Can you work these out from the model? Positions are in its coordinate system, mm. Coordinates: 2 decimals unless noted, no trailing zeros. Write each loop counter-clockwise with the first axis right and the second up, starting at its lowest first coordinate (ties: lowest second). Pieces come first, ordered by that corner, then holes. Notation, with made-up numbers: M 60,-35.5 L 75,-35.5 A18 cw 75,-26.5 Z; hole C 78.25,42.25 d6. An arc over 180 degrees is marked long. Answer as a JSON object with one key per item and string values. Group by question number.
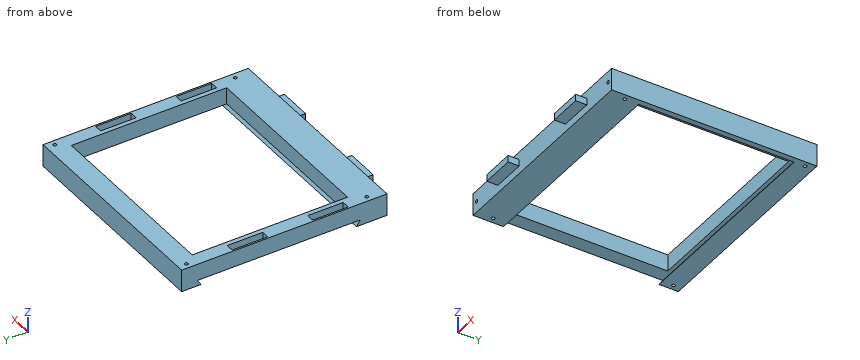
from build123d import *

# Parameters (mm, degrees)
ESBO_O1_W                = 195
ESBO_O1_H                = 185
RESSALTO_EXTRUS_O1_DEPTH = 20
ESBO_O2_W                = 30
ESBO_O2_H                = 6
RESSALTO_EXTRUS_O2_DEPTH = 10
ESBO_O3_W                = 7
ESBO_O3_H                = 32
CORTE_EXTRUS_O1_DEPTH    = 10
ESBO_O5_R                = 1.5
CORTE_EXTRUS_O3_DEPTH    = 8
ESBO_O6_R                = 1.5
CORTE_EXTRUS_O4_DEPTH    = 21
ESBO_O8_W                = 170
ESBO_O8_H                = 140
CORTE_EXTRUS_O6_DEPTH    = 21
CORTE_EXTRUS_O7_DEPTH    = 190


with BuildPart() as part:
    # Esboço1 → Ressalto-extrusão1 (new body)
    with BuildSketch(Plane.XY):
        Rectangle(ESBO_O1_W, ESBO_O1_H)
    extrude(amount=RESSALTO_EXTRUS_O1_DEPTH)

    # Esboço2 → Ressalto-extrusão2 (add)
    with BuildSketch(Plane.XZ.offset(92.5)):
        with Locations((-47.5, 10)):
            Rectangle(ESBO_O2_W, ESBO_O2_H)
        with Locations((47.5, 10)):
            Rectangle(ESBO_O2_W, ESBO_O2_H)
    extrude(amount=RESSALTO_EXTRUS_O2_DEPTH)

    # Esboço3 → Corte-extrusão1 (cut)
    with BuildSketch(Plane.XY.offset(20)):
        with Locations((-92.5, 30)):
            Rectangle(ESBO_O3_W, ESBO_O3_H)
        with Locations((-92.5, -42.5)):
            Rectangle(ESBO_O3_W, ESBO_O3_H)
        with Locations((92.5, -42.5)):
            Rectangle(ESBO_O3_W, ESBO_O3_H)
        with Locations((92.5, 30)):
            Rectangle(ESBO_O3_W, ESBO_O3_H)
    extrude(amount=-CORTE_EXTRUS_O1_DEPTH, mode=Mode.SUBTRACT)

    # Esboço5 → Corte-extrusão3 (cut)
    with BuildSketch(Plane.XZ.offset(92.5)):
        with Locations((-92.5, 10)):
            Circle(ESBO_O5_R)
        with Locations((92.5, 10)):
            Circle(ESBO_O5_R)
    extrude(amount=-CORTE_EXTRUS_O3_DEPTH, mode=Mode.SUBTRACT)

    # Esboço6 → Corte-extrusão4 (cut, through all)
    with BuildSketch(Plane(origin=(0, 0, 0), x_dir=(-1, 0, 0), z_dir=(0, 0, -1))):
        with Locations((-92.5, 85)):
            Circle(ESBO_O6_R)
        with Locations((92.5, 85)):
            Circle(ESBO_O6_R)
        with Locations((-92.5, -77.5)):
            Circle(ESBO_O6_R)
        with Locations((92.5, -77.5)):
            Circle(ESBO_O6_R)
    extrude(amount=-CORTE_EXTRUS_O4_DEPTH, mode=Mode.SUBTRACT)

    # Esboço8 → Corte-extrusão6 (cut, through all)
    with BuildSketch(Plane(origin=(0, 0, 0), x_dir=(-1, 0, 0), z_dir=(0, 0, -1))):
        with Locations((0, 5)):
            Rectangle(ESBO_O8_W, ESBO_O8_H)
    extrude(amount=-CORTE_EXTRUS_O6_DEPTH, mode=Mode.SUBTRACT)

    # Esboço9 → Corte-extrusão7 (cut)
    with BuildSketch(Plane.ZY.offset(97.5)):
        Polygon((0, -65), (0, 75), (5, 78.501037691), (5, -68.501037691), align=None)
    extrude(amount=-CORTE_EXTRUS_O7_DEPTH, mode=Mode.SUBTRACT)


solid = part.part
Q1. If we section it at B-B on x = 22.5: List the corners of the cut face in (y, z) for me, and give its area (3 significant figures).
Q2. Will these pins go through, and if not, where does the flat tip stop? pin 1 (5.5 mm diameter, centred on x = 94, z = 14, fed in from -Y); pin 2 (0.9 mm diameter, centred on x = 93, z = 9.5, fed in from -Y); pin 3 (4 mm diameter, centred on y = 41, z = 1.5, fed in from -X).
Q3. Please list where these lines run through material, in increasing order: L1, parallel to X at y = -77.5, z = 10; L2, parallel to X at y = 45.5, z = 16; L3, parallel to Y at x = 92.5, z = 13.75.
Q4. If we section it at C-C on z = 17.5: Give the number of separate pieces and of enclosed holes in the cut face, and give its area (3 significant figures).
Q5. If we section it at D-D on x = -48: List the corners of the cut face in (y, z) for me, and give its area (3 significant figures).
Q6. If we section it at A-A on y = 6: List the corners of the cut face in (x, z) for me.
Reply:
{
 "1": {"outline": "M -92.5,0 L -65,0 L -68.5,5 L -65,5 L -65,20 L -92.5,20 Z; M 75,0 L 92.5,0 L 92.5,20 L 75,20 L 75,5 L 78.5,5 Z", "area": "882 mm^2"},
 "2": {"pin 1": "y = -92.5", "pin 2": "y = -84.5", "pin 3": "x = 92.5"},
 "3": {"L1": "-97.5 to -94, -91 to 91, 94 to 97.5", "L2": "-97.5 to -96, -89 to -85, 85 to 89, 96 to 97.5", "L3": "-92.5 to -79, -76 to -58.5, -26.5 to 14, 46 to 83.5, 86.5 to 92.5"},
 "4": {"separate pieces": "1", "enclosed holes": "9", "area": "11,400 mm^2"},
 "5": {"outline": "M -102.5,7 L -92.5,7 L -92.5,0 L -65,0 L -68.5,5 L -65,5 L -65,20 L -92.5,20 L -92.5,13 L -102.5,13 Z; M 75,0 L 92.5,0 L 92.5,20 L 75,20 L 75,5 L 78.5,5 Z", "area": "942 mm^2"},
 "6": {"outline": "M -97.5,5 L -85,5 L -85,20 L -97.5,20 Z; M 85,5 L 92.5,5 L 92.5,0 L 97.5,0 L 97.5,20 L 85,20 Z"}
}
